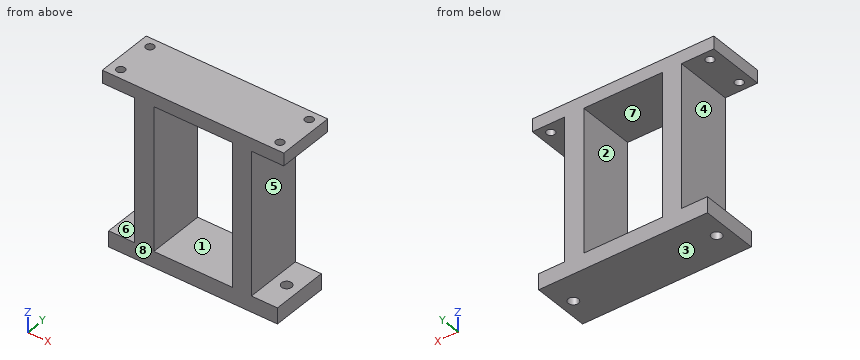
from build123d import *

# Parameters (mm, degrees)
SKETCH_1_W           = 5
SKETCH_1_H           = 18
SKETCH_1_R           = 1.3
EXTRUDE_1_DEPTH      = 4
SKETCH_2_W           = 5
SKETCH_2_H           = 18
EXTRUDE_2_DEPTH      = 54
SKETCH_3_W           = 5
SKETCH_3_H           = 18
EXTRUDE_3_DEPTH      = 53
SKETCH_4_R           = 1.6
CUT_EXTRUDE_1_DEPTH  = 50
SKETCH_8_W           = 4
SKETCH_8_H           = 18
EXTRUDE_4_DEPTH      = 53
SKETCH_9_R           = 1.3
CUT_EXTRUDE_6_DEPTH  = 12
SKETCH_14_W          = 4
SKETCH_14_H          = 18
CUT_EXTRUDE_8_DEPTH  = 5
SKETCH_15_W          = 4
SKETCH_15_H          = 18
CUT_EXTRUDE_9_DEPTH  = 5
SKETCH_16_W          = 6
SKETCH_16_H          = 18
EXTRUDE_5_DEPTH      = 45
SKETCH_17_W          = 5
SKETCH_17_H          = 18
CUT_EXTRUDE_10_DEPTH = 77
SKETCH_19_W          = 4
SKETCH_19_H          = 18
EXTRUDE_6_DEPTH      = 2


with BuildPart() as part:
    # 草图1 → 凸台-拉伸1 (new body)
    with BuildSketch(Plane.XY):
        Rectangle(SKETCH_1_W, SKETCH_1_H)
        with Locations((0, -6)):
            Circle(SKETCH_1_R, mode=Mode.SUBTRACT)
        with Locations(Location((0, 6, 0), (0, 0, 180))):
            Circle(SKETCH_1_R, mode=Mode.SUBTRACT)
    extrude_1 = extrude(amount=EXTRUDE_1_DEPTH)

    # 草图2 → 凸台-拉伸2 (add)
    with BuildSketch(Plane.XY.offset(4)):
        with Locations((-5, 0)):
            Rectangle(SKETCH_2_W, SKETCH_2_H)
    extrude_2 = extrude(amount=-EXTRUDE_2_DEPTH)

    # 草图3 → 凸台-拉伸3 (add)
    with BuildSketch(Plane.ZY.offset(7.5)):
        with Locations((-47.5, 0)):
            Rectangle(SKETCH_3_W, SKETCH_3_H)
    extrude(amount=EXTRUDE_3_DEPTH)

    # 镜向1: 凸台-拉伸2 across plane
    add(extrude_2.mirror(Plane.ZY.offset(34)))

    # 镜向2: 凸台-拉伸1 across plane
    add(extrude_1.mirror(Plane.ZY.offset(34)))

    # 草图4 → 切除-拉伸1 (cut)
    with BuildSketch(Plane(origin=(0, 0, -50), x_dir=(-1, 0, 0), z_dir=(0, 0, -1))):
        with Locations((11.5, 0)):
            Circle(SKETCH_4_R)
        with Locations((56.5, 0)):
            Circle(SKETCH_4_R)
    extrude(amount=-CUT_EXTRUDE_1_DEPTH, mode=Mode.SUBTRACT)

    # 草图8 → 凸台-拉伸4 (add)
    with BuildSketch(Plane.ZY.offset(7.5)):
        with Locations((2, 0)):
            Rectangle(SKETCH_8_W, SKETCH_8_H)
    extrude(amount=EXTRUDE_4_DEPTH)

    # 草图9 → 切除-拉伸6 (cut)
    with BuildSketch(Plane(origin=(0, 0, 0), x_dir=(-1, 0, 0), z_dir=(0, 0, -1))):
        with Locations((59, 6)):
            Circle(SKETCH_9_R)
        with Locations((59, -6)):
            Circle(SKETCH_9_R)
        with Locations((9, -6)):
            Circle(SKETCH_9_R)
        with Locations((9, 6)):
            Circle(SKETCH_9_R)
    extrude(amount=-CUT_EXTRUDE_6_DEPTH, mode=Mode.SUBTRACT)

    # 草图14 → 切除-拉伸8 (cut)
    with BuildSketch(Plane(origin=(2.5, 0, 0), x_dir=(0, 0, -1), z_dir=(1, 0, 0))):
        with Locations((-2, 0)):
            Rectangle(SKETCH_14_W, SKETCH_14_H)
    extrude(amount=-CUT_EXTRUDE_8_DEPTH, mode=Mode.SUBTRACT)

    # 草图15 → 切除-拉伸9 (cut)
    with BuildSketch(Plane.ZY.offset(70.5)):
        with Locations((2, 0)):
            Rectangle(SKETCH_15_W, SKETCH_15_H)
    extrude(amount=-CUT_EXTRUDE_9_DEPTH, mode=Mode.SUBTRACT)

    # 草图16 → 凸台-拉伸5 (add)
    with BuildSketch(Plane(origin=(0, 0, 0), x_dir=(-1, 0, 0), z_dir=(0, 0, -1))):
        with Locations((18.670705093, 0)):
            Rectangle(SKETCH_16_W, SKETCH_16_H)
        with Locations((49.329294907, 0)):
            Rectangle(SKETCH_16_W, SKETCH_16_H)
    extrude_5 = extrude(amount=EXTRUDE_5_DEPTH)

    # 草图17 → 切除-拉伸10 (cut)
    with BuildSketch(Plane.XY.offset(4)):
        with Locations((-5, 0)):
            Rectangle(SKETCH_17_W, SKETCH_17_H)
    cut_extrude_10 = extrude(amount=-CUT_EXTRUDE_10_DEPTH, mode=Mode.SUBTRACT)

    # 草图19 → 凸台-拉伸6 (add)
    with BuildSketch(Plane(origin=(-7.5, 0, 0), x_dir=(0, 0, -1), z_dir=(1, 0, 0))):
        with Locations((-2, 0)):
            Rectangle(SKETCH_19_W, SKETCH_19_H)
    extrude_6 = extrude(amount=EXTRUDE_6_DEPTH)

    # 镜向3: 凸台-拉伸5, 切除-拉伸10, 凸台-拉伸6 across plane
    add(extrude_5.mirror(Plane.ZY.offset(34)))
    add(cut_extrude_10.mirror(Plane.ZY.offset(34)), mode=Mode.SUBTRACT)
    add(extrude_6.mirror(Plane.ZY.offset(34)))


solid = part.part
The listing builds one solid part. Answer for the finished solid, in the listing's coordinates (mm). Face numbers are marked on the shaded views. A direction names the side the tool comes from. Give positions to 0.01 mm unless a question says otherwise; leave off trailing zeros. Write each loop counter-clockwise with the first axis right and the second up, starting at its lowest first coordinate (ties: lowest second). Pieces come first, ordered by that corner, then holes.
Item 1: Section A-A, the plane y = -6 is taken. Write down the section's boundary in (x, z).
Item 2: Section C-C, the plane x = -9 is taken. Write down the section's boundary in (y, z).
Item 3: Flat-ended cylindrical pins translate along their axes: P1, Ø2.5, axis at y = -2.5, z = -48, coming from the -X side; P2, Ø9, axis at y = 1, z = -31.5, coming from the -X side; P3, Ø1.9, axis at x = -56.5, y = 0, coming from the -Z side. Find the tip coordinate at first contact, or state that the pin passes through.
Item 4: Determine the mould class of the marked faces 1, 2, 3 and 4 for opening direction X: released by +X, released by -X, zero draft, split by the parting line, or undercut.
Item 5: Section B-B, the plane z = -36.5 is taken. Write down the section's boundary in (x, y).
Item 6: Section D-D, the plane x = -34 is taken. Write down the section's boundary in (y, z), plus the area to 3 significant figures.
Item 7: Which of the six approach directions +Z, -Z, +X, -X, +Y, -Y give full straight-line access (tool end or side, diameter ignored) to the marked faces 5, 6, 7 and 8?
Item 8: Find the intervals of material crossed by line 1 along Y through (x, z) = (-59, 2.25); line 2 along Z through (x, y) = (-24, -1.75); line 3 along X through (y, z) = (-7, -44), in increasing order.
Completed:
1. outline: (-62.5, 0) - (-60.3, 0) - (-60.3, 4) - (-62.5, 4) - close; (-60.5, -50) - (-7.5, -50) - (-7.5, -45) - (-15.67, -45) - (-15.67, 0) - (-10.3, 0) - (-10.3, 4) - (-57.7, 4) - (-57.7, 0) - (-52.33, 0) - (-52.33, -45) - (-60.5, -45) - close; (-7.7, 0) - (-5.5, 0) - (-5.5, 4) - (-7.7, 4) - close; hole (-46.33, -45) - (-21.67, -45) - (-21.67, 0) - (-46.33, 0) - close
2. outline: (-9, -50) - (9, -50) - (9, -45) - (-9, -45) - close; (-9, 0) - (-7.3, 0) - (-7.3, 4) - (-9, 4) - close; (-4.7, 0) - (4.7, 0) - (4.7, 4) - (-4.7, 4) - close; (7.3, 0) - (9, 0) - (9, 4) - (7.3, 4) - close
3. P1: stops at x = -60.5
3. P2: stops at x = -52.33
3. P3: stops at z = 0
4. face 1: undercut
4. face 2: undercut
4. face 3: zero draft
4. face 4: released by -X
5. outline: (-52.33, -9) - (-46.33, -9) - (-46.33, 9) - (-52.33, 9) - close; (-21.67, -9) - (-15.67, -9) - (-15.67, 9) - (-21.67, 9) - close
6. outline: (-9, -50) - (9, -50) - (9, -45) - (-9, -45) - close; (-9, 0) - (9, 0) - (9, 4) - (-9, 4) - close
6. area: 162 mm2
7. face 5: +X, +Y, -Y
7. face 6: -X, +Y, -Y
7. face 7: +Y, -Y
7. face 8: +Z, -Z, +X, -X, -Y
8. line 1: y = -9 to -7.3, -4.7 to 4.7, 7.3 to 9
8. line 2: z = -50 to -45, 0 to 4
8. line 3: x = -52.33 to -46.33, -21.67 to -15.67
